Check sheet for the drawn part. Datum: minimum x, y, z corner. Units: mm. A direction names the side the tool comes from. Coordinates: 2 decimals unless noted, no trailing zeros. Order: outer loops, then holes, each group sorted by start corner. A loop starts at its lowest first (then second) coordinate and runs counter-clockwise, first axis right, second up.
1. Cross-section at A-A (x = 33.25). Enter the section's corners in (y, z).
2. Draft check along Z on the marked faces 3, 4, 5 and 6. Enter one of: released by +Z, released by -Z, zero draft, split by the parting line, or undercut.
3. Gauge pin test, flat end, axial feed: pin 1 Ø4 at (x, z) = (19.5, 8) entering from +Y. Record the tip position at first contact, or that the pin passes through.
4. Set-up check for the marked faces 1 and 2: record each of +Z, -Z, +X, -X, +Y, -Y from which the full face is reachable in a straight line by a thin tool's end or side.
5. Cross-section at C-C (y = 6.5). Enter the section's corners in (x, z), then the cut area to 4 significant figures.
6. Thickness scan on line 1 (Z direction, x = 17.5, y = 5.5); line 2 (X direction, y = 1.6, z = 10.5); line 3 (Z direction, x = 33.25, y = 1.15). Record the ranges inside material, lowest first.
7. Cross-section at B-B (z = 10.5). Enter the section's corners in (x, y), then the cut area to 3 significant figures.
8. Cross-section at D-D (z = 37.5). Enter the section's corners in (x, y), then the cut area to 3 significant figures.
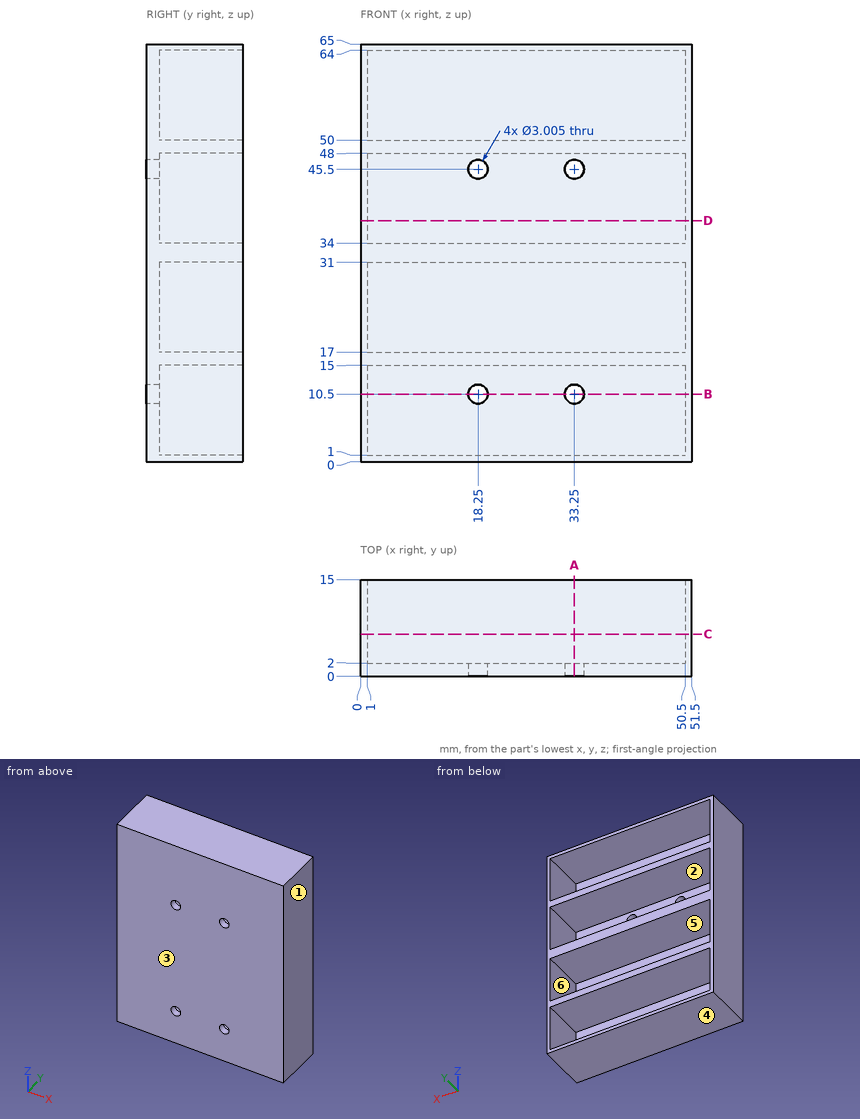
Data:
1. outline: (0, 0) - (15, 0) - (15, 1) - (2, 1) - (2, 9) - (0, 9) - close; (0, 12) - (2, 12) - (2, 15) - (15, 15) - (15, 17) - (2, 17) - (2, 31) - (15, 31) - (15, 34) - (2, 34) - (2, 44) - (0, 44) - close; (0, 47) - (2, 47) - (2, 48) - (15, 48) - (15, 50) - (2, 50) - (2, 64) - (15, 64) - (15, 65) - (0, 65) - close
2. face 3: zero draft
2. face 4: released by -Z
2. face 5: undercut
2. face 6: undercut
3. pin 1: stops at y = 2
4. face 1: +Z, -Z, +X, +Y, -Y
4. face 2: +Y
5. outline: (0, 0) - (51.5, 0) - (51.5, 65) - (0, 65) - close; hole (1, 1) - (50.5, 1) - (50.5, 15) - (1, 15) - close; hole (1, 17) - (50.5, 17) - (50.5, 31) - (1, 31) - close; hole (1, 34) - (50.5, 34) - (50.5, 48) - (1, 48) - close; hole (1, 50) - (50.5, 50) - (50.5, 64) - (1, 64) - close
5. area: 575.5 mm2
6. line 1: z = 0 to 1, 15 to 17, 31 to 34, 48 to 50, 64 to 65
6. line 2: x = 0 to 16.75, 19.75 to 31.75, 34.75 to 51.5
6. line 3: z = 0 to 9, 12 to 44, 47 to 65
7. outline: (0, 0) - (16.75, 0) - (16.75, 2) - (1, 2) - (1, 15) - (0, 15) - close; (19.75, 0) - (31.75, 0) - (31.75, 2) - (19.75, 2) - close; (34.75, 0) - (51.5, 0) - (51.5, 15) - (50.5, 15) - (50.5, 2) - (34.75, 2) - close
7. area: 117 mm2
8. outline: (0, 0) - (51.5, 0) - (51.5, 15) - (50.5, 15) - (50.5, 2) - (1, 2) - (1, 15) - (0, 15) - close
8. area: 129 mm2
